Could you check a few things on this model? Use its own coordinates, in mm. A direction names the side the tool comes from. Coordinates: 2 decimals unless noted, no trailing zeros. Loops run counter-clockwise (first coordinate to the right, second up) from the corner with the lowest first, then second, coordinate; pieces in that order, holes last. Notation, with made-up numbers: (5, 24) - (31, 24) arc R13 cw to (31, 30) - close; hole circle Ø3 at (65.25, 21). An arc over 180 degrees is marked (long way). One line per question, with ' | ' between items. Start each with the question number.
1. Please list where these lines run through material, in increasing order: L1, parallel to X at y = 35.5, z = 50; L2, parallel to X at y = 6, z = 75; L3, parallel to Z at x = 185, y = 10.5. Write a range as [from, to].
2. I want a section at C-C, the plane z = 84.5. Write out the boundary of the cut face in (x, y).
3. I want a section at D-D, the plane z = 50. Write out the boundary of the cut face in (x, y), then the cut area to 3 significant figures.
4. I want a section at A-A, the plane y = 27. Write out the boundary of the cut face in (x, z).
5. Which directions (+Z, -Z, +X, -X, +Y, -Y) give clear straight access to the entire face, cutting with the end or side of a thin tool? Please do faces 1 (the cylindrical face through (27, 81, 50)), 2 (the flat face through (171, 63.5, 50)), 3 (the flat face through (160, 40, 27.5)), 4 (the flat face through (160, 40, 72.5)), 5 (the flat face through (117, 35, 49)).
6. We'd pull the mould along X, two halves only. Please class faces 6 (the cylindrical face through (207.495, 40.432, 50.495)), 7 (the flat face through (63, 81, 59)), 8 (the flat face through (195, 0, 49)): pulls with the +X half, pulls with the -X half, needs draft (parallel to the pull), parting line crosses it, or undercut.
7. I'm going to push flat-ended pins straight in: P1, Ø14.5, axis at x = 185, z = 50, coming from the +Y side; P2, Ø5, axis at x = 174, y = 32, coming from the -Z side; P3, Ø10, axis at x = 70.5, z = 69.5, coming from the -Y side; P4, Ø10, axis at y = 34, z = 43.5, coming from the +X side. Where does each tip first touch, or does it pass through?
8. I want a section at B-B, the plane y = 10. Write out the boundary of the cut face in (x, z), then the cut area to 3 significant figures.
from build123d import *

# Parameters (mm, degrees)
BOSS_EXTRUDE1_DEPTH = 100
CUT_EXTRUDE1_DEPTH  = 100
BOSS_EXTRUDE2_DEPTH = 45.5
HOLE1_D             = 18
HOLE2_D             = 18
HOLE2_DEPTH         = 18


with BuildPart() as part:
    # Sketch1 → Boss-Extrude1 (new body)
    with BuildSketch(Plane.XY):
        Polygon((0, 0), (0, 90), (135, 90), (135, 18), (270, 18), (270, 0), (117, 0), (117, 72), (18, 72), (18, 0), align=None)
    extrude(amount=BOSS_EXTRUDE1_DEPTH)

    # Sketch2 → Cut-Extrude1 (cut)
    with BuildSketch(Plane(origin=(0, 90, 0), x_dir=(1, 0, 0), z_dir=(0, 1, 0))):
        with BuildLine():
            Line((36, -41), (90, -41))
            ThreePointArc((90, -41), (99, -50), (90, -59))
            Line((90, -59), (36, -59))
            ThreePointArc((36, -59), (27, -50), (36, -41))
        make_face()
    extrude(amount=-CUT_EXTRUDE1_DEPTH, mode=Mode.SUBTRACT)

    # Sketch4 → Boss-Extrude2 (add)
    with BuildSketch(Plane(origin=(0, 18, 0), x_dir=(1, 0, 0), z_dir=(0, 1, 0))):
        with BuildLine():
            Line((185, -27.5), (135, -27.5))
            Line((135, -27.5), (135, -72.5))
            Line((135, -72.5), (185, -72.5))
            ThreePointArc((185, -72.5), (207.5, -50), (185, -27.5))
        make_face()
    extrude(amount=BOSS_EXTRUDE2_DEPTH)

    # Hole1 (through all)
    with Locations(Plane(origin=(0, 63.5, 0), x_dir=(1, 0, 0), z_dir=(0, 1, 0))):
        with Locations((185, -50)):
            Hole(HOLE1_D / 2)

    # Hole2
    with Locations(Plane.ZY):
        with Locations((55, 27)):
            Hole(HOLE2_D / 2, depth=HOLE2_DEPTH)


solid = part.part
Results are:
1) L1: x = [0, 18], [117, 176], [194, 207.5] | L2: x = [0, 18], [117, 270] | L3: z = [0, 41], [59, 100]
2) outline: (0, 0) - (18, 0) - (18, 72) - (117, 72) - (117, 0) - (270, 0) - (270, 18) - (135, 18) - (135, 90) - (0, 90) - close
3) outline: (0, 0) - (18, 0) - (18, 19.52) - (0, 19.52) - close; (0, 34.48) - (18, 34.48) - (18, 72) - (27, 72) - (27, 90) - (0, 90) - close; (99, 72) - (117, 72) - (117, 0) - (176, 0) - (176, 63.5) - (135, 63.5) - (135, 90) - (99, 90) - close; (194, 0) - (270, 0) - (270, 18) - (207.5, 18) - (207.5, 63.5) - (194, 63.5) - close | area: 8,040 mm2
4) outline: (0, 0) - (18, 0) - (18, 46) - (0, 46) - close; (0, 64) - (18, 64) - (18, 100) - (0, 100) - close; (117, 0) - (135, 0) - (135, 27.5) - (185, 27.5) arc R22.5 ccw to (185, 72.5) - (135, 72.5) - (135, 100) - (117, 100) - close; hole circle Ø18 at (185, 50)
5) face 1: +Y, -Y | face 2: +Z, -Z, +X, +Y | face 3: -Z, +X, +Y | face 4: +Z, +X, +Y | face 5: +Z, -Z, -Y
6) face 6: pulls with the +X half | face 7: undercut | face 8: needs draft
7) P1: passes through | P2: stops at z = 27.5 | P3: stops at y = 72 | P4: stops at x = 207.45
8) outline: (0, 0) - (18, 0) - (18, 100) - (0, 100) - close; (117, 0) - (270, 0) - (270, 100) - (117, 100) - close; hole circle Ø18 at (185, 50) | area: 16,800 mm2
